Autodesk Inventor part; units mm, degrees
ref_plane "YZ Plane" through (0, 0, 0) normal (1, 0, 0) x (0, 1, 0)
ref_plane "XZ Plane" through (0, 0, 0) normal (0, 1, 0) x (-1, 0, 0)
ref_plane "XY Plane" through (0, 0, 0) normal (0, 0, 1) x (1, 0, 0)
sketch "Sketch1" plane through (0, 0, 0) normal (0, 0, 1) x (1, 0, 0)
  line L0 (0, 0) -> (88.9, 0)
  line L1 (88.9, 0) -> (88.9, 228.6)
  line L2 (88.9, 228.6) -> (0, 228.6)
  line L3 (0, 228.6) -> (0, 0)
  dimension "d0" = 88.9
  dimension "d1" = 228.6
extrude "door" add sketch "Sketch1" along normal mid plane 22.86
sketch "Sketch2" plane through (0, 0, 0) normal (0, 0, 1) x (1, 0, 0)
  line L0 (88.9, 228.6) -> (0, 228.6)
  line L1 (88.9, 0) -> (0, 0)
  line L2 (4.4901, 64.0899) -> (4.4901, 50.2101)
  line L3 (4.4901, 50.2101) -> (0, 45.72)
  line L4 (0, 45.72) -> (-4.4901, 41.2299)
  line L5 (-4.4901, 41.2299) -> (-4.4901, 27.3501)
  line L6 (-4.4901, 27.3501) -> (0, 22.86)
  line L7 (0, 22.86) -> (0, 45.72)
  line L8 (0, 22.86) -> (4.4901, 18.3699)
  line L9 (4.4901, 18.3699) -> (4.4901, 4.4901)
  line L10 (4.4901, 4.4901) -> (0, 0)
  line L11 (0, 0) -> (0, 22.86)
  line L12 (0, 45.72) -> (0, 68.58)
  line L13 (-4.4901, 178.3899) -> (-4.4901, 164.5101)
  line L14 (0, 160.02) -> (0, 182.88)
  line L15 (-4.4901, 164.5101) -> (0, 160.02)
  line L16 (0, 160.02) -> (4.4901, 155.5299)
  line L17 (4.4901, 155.5299) -> (4.4901, 141.6501)
  line L18 (4.4901, 141.6501) -> (0, 137.16)
  line L19 (0, 137.16) -> (0, 160.02)
  line L20 (0, 137.16) -> (-4.4901, 132.6699)
  line L21 (-4.4901, 132.6699) -> (-4.4901, 118.7901)
  line L22 (0, 114.3) -> (0, 137.16)
  line L23 (-4.4901, 118.7901) -> (0, 114.3)
  line L24 (0, 114.3) -> (4.4901, 109.8099)
  line L25 (-4.4901, 73.0701) -> (0, 68.58)
  line L26 (-4.4901, 86.9499) -> (-4.4901, 73.0701)
  line L27 (0, 68.58) -> (0, 91.44)
  line L28 (0, 91.44) -> (-4.4901, 86.9499)
  line L29 (4.4901, 95.9301) -> (0, 91.44)
  line L30 (4.4901, 109.8099) -> (4.4901, 95.9301)
  line L31 (0, 91.44) -> (0, 114.3)
  line L32 (0, 68.58) -> (4.4901, 64.0899)
  line L33 (0, 228.6) -> (-4.4901, 224.1099)
  line L34 (0, 182.88) -> (-4.4901, 178.3899)
  line L35 (4.4901, 187.3701) -> (0, 182.88)
  line L36 (4.4901, 201.2499) -> (4.4901, 187.3701)
  line L37 (0, 182.88) -> (0, 205.74)
  line L38 (0, 205.74) -> (4.4901, 201.2499)
  line L39 (-4.4901, 210.2301) -> (0, 205.74)
  line L40 (-4.4901, 224.1099) -> (-4.4901, 210.2301)
  line L41 (0, 205.74) -> (0, 228.6)
  point P0 (-4.4901, 34.29)
  point P1 (4.4901, 57.15)
  point P2 (-4.4901, 80.01)
  point P3 (4.4901, 102.87)
  point P4 (-4.4901, 125.73)
  point P5 (4.4901, 148.59)
  point P6 (-4.4901, 171.45)
  point P7 (4.4901, 194.31)
  point P8 (-4.4901, 217.17)
  dimension "d36" = 6.35
  dimension "d37" = 228.6
  dimension "d38" = 11.43
  dimension "d39" = 11.43
  dimension "d40" = 11.43
  dimension "d41" = 11.43
  dimension "d42" = 11.43
  dimension "d43" = 11.43
  dimension "d44" = 11.43
  dimension "d45" = 11.43
  dimension "d46" = 45
  dimension "d47" = 45
extrude "teeth cut" cut sketch "Sketch2" along normal mid plane 17.78 contours L8 L9 L10 L11 | L37 L38 L36 L35 | L19 L16 L17 L18 | L31 L24 L30 L29 | L2 L3 L12 L32
extrude "teeth make" add sketch "Sketch2" along normal mid plane 17.78 contours L7 L6 L5 L4 | L39 L40 L33 L41 | L15 L13 L34 L14 | L23 L21 L20 L22 | L25 L26 L28 L27
equation "\"d21\" = d19"
equation "\"d48\" = 0.05 * d37"
properties part number "door (right side) 2nd map"
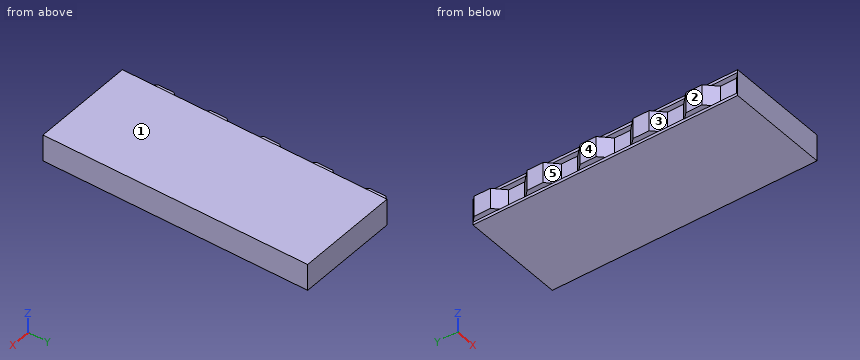
The listing builds one solid part. Answer for the finished solid, in the listing's coordinates (mm). Face numbers are marked on the shaded views. A direction names the side the tool comes from. Round coordinates to 2 decimals unless told otherwise and drop trailing zeros. Order: outer loops, then holes, each group sorted by start corner. A loop starts at its lowest first (then second) coordinate and runs counter-clockwise, first axis right, second up. Notation, with made-up numbers: (30.25, 68.5) - (41.25, 68.5) arc R22 ccw to (41.25, 77.5) - close; hole circle Ø3 at (-18, 53.5). An arc over 180 degrees is marked (long way). Write item = value, one per line. Start each with the question number.
1) For a pull along Z with two mould halves and no side action, classify the marked faces 1, 2 and 3 as released by +Z, released by -Z, zero draft, split by the parting line, or undercut.
2) Section A-A, the plane y = 196.5 is taken. Write down the section's boundary in (x, z), plus the area to 3 significant figures.
3) Section B-B, the plane z = -3.5 is taken. Write down the section's boundary in (x, y).
4) Given pin 1 (1.3 mm diameter, centred on x = -1, y = 213, fed in from +Z); pin 2 (0.8 mm diameter, centred on y = 84, z = -10, fed in from -X); pin 3 (2 mm diameter, centred on x = -2.5, y = 30, fed in from -Z), each flat-ended and moving along its own axis, determine where each tip first touches the part or whether it passes through.
5) For the marked faces 4 and 5, determine the directions among +Z, -Z, +X, -X, +Y, -Y from which every point of the face is accessible in a straight line to the end or side of a thin tool.
6) Straight lines are drawn through the part: L1, parallel to Y at x = 0.5, z = 5.75; L2, parallel to X at y = 12, z = -6.5; L3, parallel to X at y = 108.5, z = -9.75. For each, find the intervals that lie inside material, in ascending order.
Results list:
q1.face_1 = released by +Z
q1.face_2 = zero draft
q1.face_3 = undercut
q2.outline = (0, -11.43) - (88.9, -11.43) - (88.9, 11.43) - (0, 11.43) - (0, 8.89) - (4.49, 8.89) - (4.49, -8.89) - (0, -8.89) - close
q2.area = 1,950 mm^2
q3.outline = (-4.49, 27.35) - (4.49, 18.37) - (4.49, 4.49) - (0, 0) - (88.9, 0) - (88.9, 228.6) - (0, 228.6) - (-4.49, 224.11) - (-4.49, 210.23) - (4.49, 201.25) - (4.49, 187.37) - (-4.49, 178.39) - (-4.49, 164.51) - (4.49, 155.53) - (4.49, 141.65) - (-4.49, 132.67) - (-4.49, 118.79) - (4.49, 109.81) - (4.49, 95.93) - (-4.49, 86.95) - (-4.49, 73.07) - (4.49, 64.09) - (4.49, 50.21) - (-4.49, 41.23) - close
q4.pin_1 = 8.89
q4.pin_2 = 0
q4.pin_3 = -8.89
q5.face_4 = +Z, -Z, -X, +Y, -Y
q5.face_5 = -X
q6.L1 = 0 to 0.5, 22.36 to 46.22, 68.08 to 91.94, 113.8 to 137.66, 159.52 to 183.38, 205.24 to 228.6
q6.L2 = 4.49 to 88.9
q6.L3 = 0 to 88.9
